The listing builds one solid part. Answer for the finished solid, in the listing's coordinates (mm). Give positions to 0.01 mm unless a question says otherwise; leave off trailing zeros. Answer as CSV lines item,"result". Start each with the question number.
1. Consider line 1 along X through (y, z) = (29, -2.5); line 2 along X through (y, z) = (11.5, 0.5); line 3 along Y through (x, z) = (27, 2). Determine where each line is inside the solid, lowest interval first. Write a range as [from, to].
2. Flat-ended cylindrical pins translate along their axes: pin 1 (1.5 mm diameter, centred on y = 6.5, z = -3.5, fed in from -X); pin 2 (12 mm diameter, centred on x = -11.5, y = 35.5, fed in from -Z); pin 3 (3 mm diameter, centred on x = 7.5, z = 3.5, fed in from +Y); pin 4 (8 mm diameter, centred on x = -5.5, y = 34, fed in from +Z). Find the tip coordinate at first contact, or state that the pin passes through.
3. Determine the mould class of faces 1 (the flat face through (-1, 0, 0)), 2 (the conical face through (33.02, 25.64, 0.14)), 3 (the conical face through (-31.37, 21.4, 1.15)) for opening direction Y: +Y half, -Y half, draft (parallel to the pull), parting line (faces both ways), or undercut.
from build123d import *

# Parameters (mm, degrees)
SKETCH1_W           = 100
SKETCH1_H           = 10
BOSS_EXTRUDE1_DEPTH = 50
BOSS_EXTRUDE1_TAPER = 3
FILLET1_R           = 2
SKETCH2_R           = 16
CUT_EXTRUDE1_DEPTH  = 50
SKETCH3_R           = 2
CUT_EXTRUDE2_DEPTH  = 105
CUT_EXTRUDE2_DRAFT  = -1


with BuildPart() as part:
    # Sketch1 → Boss-Extrude1 (new body)
    with BuildSketch(Plane(origin=(0, 0, 0), x_dir=(1, 0, 0), z_dir=(0, 1, 0))):
        Rectangle(SKETCH1_W, SKETCH1_H)
    extrude(amount=BOSS_EXTRUDE1_DEPTH, taper=BOSS_EXTRUDE1_TAPER)

    # Fillet1
    fillet1_edges = [part.edges().sort_by_distance(p)[0] for p in [
        (0, 50, 2.379611036),
        (0, 50, -2.379611036),
    ]]
    fillet(fillet1_edges, radius=FILLET1_R)

    # Sketch2 → Cut-Extrude1 (cut)
    with BuildSketch(Plane(origin=(0, 0.261321158, -4.986304738), x_dir=(-1, 0, 0), z_dir=(0, 0.052335956242943876, -0.998629534754574))):
        with Locations(Location((-1.376828388, 24.738320219, 0), (0, 0, 90))):
            Circle(SKETCH2_R)
    extrude(amount=-CUT_EXTRUDE1_DEPTH, mode=Mode.SUBTRACT)


with BuildPart() as cut_extrude2_tool:
    # Sketch3 → Cut-Extrude2 (with draft: the straight prism first)
    with BuildSketch(Plane(origin=(49.863047384, 2.613211582, 0), x_dir=(0, 0, -1), z_dir=(0.998629534754574, 0.052335956242943876, 0))):
        with Locations((-1.067678457, 22.417510838)):
            Circle(SKETCH3_R)
    extrude(amount=-CUT_EXTRUDE2_DEPTH)
    # Cut-Extrude2: the draft: its side faces are tilted about the plane it starts from
    cut_extrude2_sides = [cut_extrude2_tool.faces().sort_by_distance(p)[0] for p in [
        (-3.738245057, 22.252362297, 3.067678457),
    ]]
    draft(cut_extrude2_sides, Plane(origin=(49.863047384, 2.613211582, 0), x_dir=(0, 0, -1), z_dir=(0.998629534754574, 0.052335956242943876, 0)), CUT_EXTRUDE2_DRAFT)


with BuildPart() as part_1:
    add(part.part)

    # Cut-Extrude2: cut by cut_extrude2_tool
    add(cut_extrude2_tool.part, mode=Mode.SUBTRACT)


solid = part_1.part
Checks:
1,line 1,"x = [-48.48, -14.09], [16.84, 48.48]"
1,line 2,"x = [-49.4, -7.62], [10.38, 49.4]"
1,line 3,"y = [0, 22.54], [25.19, 49.3]"
2,pin 1,"stops at x = -49.7"
2,pin 2,"stops at z = -3.43"
2,pin 3,"stops at y = 49.3"
2,pin 4,"passes through"
3,face 1,"-Y half"
3,face 2,"undercut"
3,face 3,"undercut"
